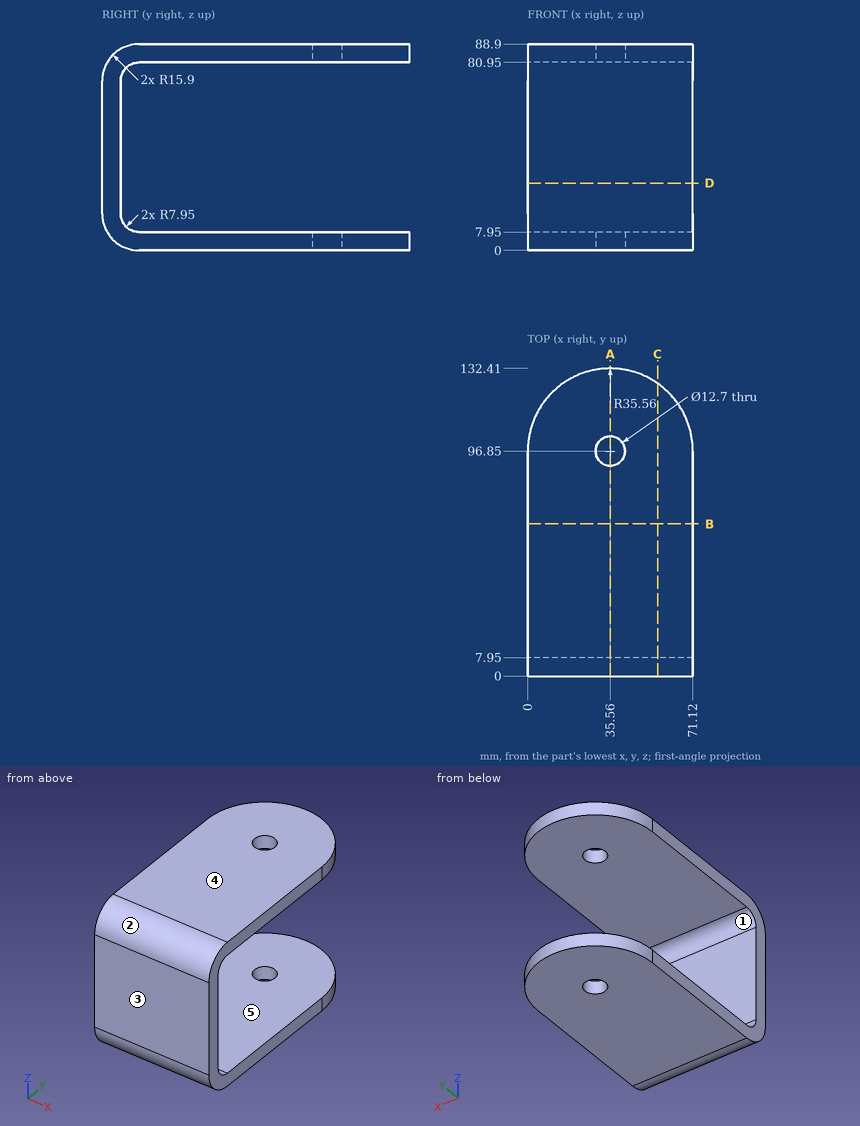
Print and shaded views of the part. All mm, measured from the part's lowest x, y and z. A direction names the side the tool comes from. Coordinates: 2 decimals unless noted, no trailing zeros. Loops run counter-clockwise (first coordinate to the right, second up) from the corner with the lowest first, then second, coordinate; pieces in that order, holes last. Notation, with made-up numbers: (67.5, -31.5) -> (104.5, -31.5) arc R19 ccw to (104.5, -20.5) -> close; hole circle Ø5 at (-34.75, 53.5). An arc over 180 degrees is marked (long way). Use a Markdown table: item, result. Add a question column.
Item 1: Band-saw the part on C-C on x = 56. Write the cut outline in (y, z), plus the area to 3 significant figures.
Item 2: Band-saw the part on B-B on y = 65.5. Write the cut outline in (x, z), plus the area to 3 significant figures.
Item 3: Pull direction Z, two halves, no side cores. Call the marked faces 3, 4 and 5: +Z half, -Z half, draft (parallel to the pull), parting line (faces both ways), or undercut.
Item 4: Which spindle directions (+Z, -Z, +X, -X, +Y, -Y) get a long thin tool onto all of the face, cutting with end or side? Do the marked faces 1 and 2. Say none if no direction does.
Item 5: Band-saw the part on D-D on z = 29. Write the cut outline in (x, y).
Item 6: Probe probe 1 along Z at (x, y) = (38.5, 76.5); probe 2 along Y at (x, z) = (57, 19.5); probe 3 along X at (y, z) = (102, 82) (1 decimal). List the from-to ranges inside material, lowest first.
Item 7: Band-saw the part on A-A on x = 35.56. Write the cut outline in (y, z).
Item 8: Flat gauge pin, fed straight in: P1, Ø8, axis at x = 45, z = 25.5, coming from the +Y side. Where does the tip first touch, or does it go through?
Geometry says:
| question | item | result |
|---|---|---|
| 1 | outline | (0, 15.9) arc R15.9 ccw to (15.9, 0) -> (125.95, 0) -> (125.95, 7.95) -> (15.9, 7.95) arc R7.95 cw to (7.95, 15.9) -> (7.95, 73) arc R7.95 cw to (15.9, 80.95) -> (125.95, 80.95) -> (125.95, 88.9) -> (15.9, 88.9) arc R15.9 ccw to (0, 73) -> close |
| 1 | area | 2,500 mm² |
| 2 | outline | (0, 0) -> (71.12, 0) -> (71.12, 7.95) -> (0, 7.95) -> close; (0, 80.95) -> (71.12, 80.95) -> (71.12, 88.9) -> (0, 88.9) -> close |
| 2 | area | 1,130 mm² |
| 3 | face 3 | draft |
| 3 | face 4 | +Z half |
| 3 | face 5 | undercut |
| 4 | face 1 | +X, -X, +Y |
| 4 | face 2 | +Z, +X, -X, -Y |
| 5 | outline | (0, 0) -> (71.12, 0) -> (71.12, 7.95) -> (0, 7.95) -> close |
| 6 | probe 1 | 0 to 7.95, 80.95 to 88.9 |
| 6 | probe 2 | 0 to 7.95 |
| 6 | probe 3 | 0.4 to 31.8, 39.3 to 70.7 |
| 7 | outline | (0, 15.9) arc R15.9 ccw to (15.9, 0) -> (90.5, 0) -> (90.5, 7.95) -> (15.9, 7.95) arc R7.95 cw to (7.95, 15.9) -> (7.95, 73) arc R7.95 cw to (15.9, 80.95) -> (90.5, 80.95) -> (90.5, 88.9) -> (15.9, 88.9) arc R15.9 ccw to (0, 73) -> close; (103.2, 0) -> (132.41, 0) -> (132.41, 7.95) -> (103.2, 7.95) -> close; (103.2, 80.95) -> (132.41, 80.95) -> (132.41, 88.9) -> (103.2, 88.9) -> close |
| 8 | P1 | y = 7.95 |
